CAD build for the part. Positions are in the model's coordinates, mm. Coordinates: 2 decimals unless noted, no trailing zeros. Order: outer loops, then holes, each group sorted by start corner. A loop starts at its lowest first (then second) coordinate and runs counter-clockwise, first axis right, second up. Notation, with made-up numbers: (10, 57.5) - (47, 57.5) arc R17 ccw to (47, 68.5) - close; hole circle Ø11 at (52.5, 40.5). An arc over 180 degrees is marked (long way). Write each question's results on one line, items separated by ' | '. Start each with the question number.
Q1. Band-saw the part on A-A, the plane x = 0. Write the cut outline in (y, z).
Q2. Band-saw the part on D-D, the plane x = 22. Write the cut outline in (y, z).
Q3. Wall check: probe 1 along Z at (x, y) = (0, -5.5); probe 2 along Z at (x, y) = (9.5, -7); probe 3 along Z at (x, y) = (14.5, -2.75). Give the ranges that are in metal, low to high.
Q4. Pin check, flat tips, straight feed: P1, Ø2.5, axis at x = -15, z = 0, coming from the -Y side; P2, Ø3, axis at x = 11, y = -5, coming from the -Z side; P3, Ø5, axis at y = -1, z = -10.5, coming from the +X side; P4, Ø1.5, axis at y = -7.5, z = -22, coming from the +X side. Stop position of each tip, or through.
Q5. Band-saw the part on C-C, the plane y = -3.5. Count the separate pieces of the cut face and the enclosed holes in it, then the cut area to 3 significant figures.
Q6. Band-saw the part on B-B, the plane z = 0. Write the cut outline in (x, y).
```python
from build123d import *

# Parameters (mm, degrees)
F0_R     = 31.59
F0_R_2   = 1.5
F0_R_3   = 2.5
F1_DEPTH = 9.55


with BuildPart() as f1:
    # F0 (on Front) → F1 (new body)
    with BuildSketch(Plane.XZ):
        Circle(F0_R)
        with Locations((-8.55, -8.55)):
            Circle(F0_R_2, mode=Mode.SUBTRACT)
        with Locations((0, -22)):
            Circle(F0_R_2, mode=Mode.SUBTRACT)
        with Locations((0, -15)):
            Circle(F0_R_2, mode=Mode.SUBTRACT)
        with Locations((8.55, -8.55)):
            Circle(F0_R_2, mode=Mode.SUBTRACT)
        with Locations((-22, 0)):
            Circle(F0_R_2, mode=Mode.SUBTRACT)
        with Locations((-15, 0)):
            Circle(F0_R_2, mode=Mode.SUBTRACT)
        with Locations((-8.55, 8.55)):
            Circle(F0_R_2, mode=Mode.SUBTRACT)
        Circle(F0_R_3, mode=Mode.SUBTRACT)
        with Locations((15, 0)):
            Circle(F0_R_2, mode=Mode.SUBTRACT)
        with Locations((0, 15)):
            Circle(F0_R_2, mode=Mode.SUBTRACT)
        with Locations((8.55, 8.55)):
            Circle(F0_R_2, mode=Mode.SUBTRACT)
        with Locations((22, 0)):
            Circle(F0_R_2, mode=Mode.SUBTRACT)
        with Locations((0, 22)):
            Circle(F0_R_2, mode=Mode.SUBTRACT)
    extrude(amount=F1_DEPTH)


solid = f1.part
```
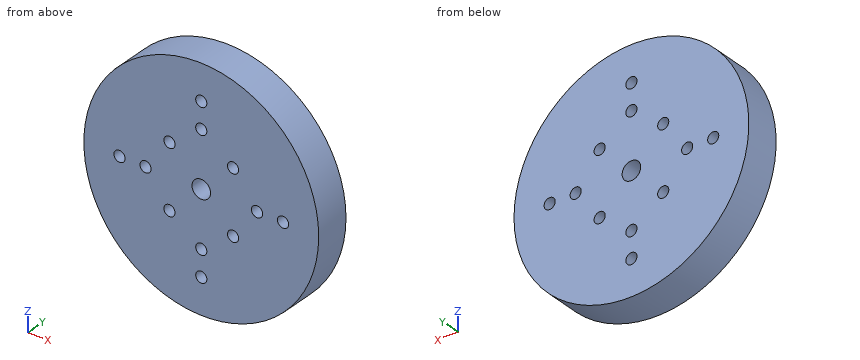
Results below:
1) outline: (-9.55, -31.59) - (0, -31.59) - (0, -23.5) - (-9.55, -23.5) - close; (-9.55, -20.5) - (0, -20.5) - (0, -16.5) - (-9.55, -16.5) - close; (-9.55, -13.5) - (0, -13.5) - (0, -2.5) - (-9.55, -2.5) - close; (-9.55, 2.5) - (0, 2.5) - (0, 13.5) - (-9.55, 13.5) - close; (-9.55, 16.5) - (0, 16.5) - (0, 20.5) - (-9.55, 20.5) - close; (-9.55, 23.5) - (0, 23.5) - (0, 31.59) - (-9.55, 31.59) - close
2) outline: (-9.55, -22.67) - (0, -22.67) - (0, -1.5) - (-9.55, -1.5) - close; (-9.55, 1.5) - (0, 1.5) - (0, 22.67) - (-9.55, 22.67) - close
3) probe 1: z = -31.59 to -23.5, -20.5 to -16.5, -13.5 to -2.5, 2.5 to 13.5, 16.5 to 20.5, 23.5 to 31.59 | probe 2: z = -30.13 to -9.71, -7.39 to 7.39, 9.71 to 30.13 | probe 3: z = -28.07 to -1.41, 1.41 to 28.07
4) P1: passes through | P2: stops at z = -30.13 | P3: stops at x = 30.56 | P4: stops at x = 23.37
5) separate pieces: 1 | enclosed holes: 13 | area: 3,030 mm²
6) outline: (-31.59, -9.55) - (-23.5, -9.55) - (-23.5, 0) - (-31.59, 0) - close; (-20.5, -9.55) - (-16.5, -9.55) - (-16.5, 0) - (-20.5, 0) - close; (-13.5, -9.55) - (-2.5, -9.55) - (-2.5, 0) - (-13.5, 0) - close; (2.5, -9.55) - (13.5, -9.55) - (13.5, 0) - (2.5, 0) - close; (16.5, -9.55) - (20.5, -9.55) - (20.5, 0) - (16.5, 0) - close; (23.5, -9.55) - (31.59, -9.55) - (31.59, 0) - (23.5, 0) - close
